```python
from build123d import *
from build123d import SkipClean  # not in build123d's __all__

# Parameters (mm, degrees)
F0_R          = 31.75
F1_DEPTH      = 2.54
F2_R          = 27.305
F2_R_2        = 22.225
F2_R_3        = 6.985
F3_DEPTH      = 5.08
F4_R          = 4.1275
F5_DEPTH      = 25.4
F5_DEPTH_BACK = 96
F7_DEPTH      = 25.4
F7_DEPTH_BACK = 5.081
F8_T1_DEPTH   = 2.54
F10_DEPTH     = 25.4


# Not quite as in the source:
# - a fillet or chamfer that OpenCascade refuses, or shapes differently, is made with other operations: its cross-section is extruded or revolved along the edge and cut away or added
# - an extrude ends at something that could not be found from the text; its depth is read off the source's solid


with BuildPart() as f1:
    # F0 (on Top) → F1 (new body)
    with BuildSketch(Plane.XY):
        Circle(F0_R)
    extrude(amount=F1_DEPTH)

    # F2 (on face) → F3 (join)
    with BuildSketch(Plane.XY.offset(2.54)):
        Circle(F2_R)
        Circle(F2_R_2, mode=Mode.SUBTRACT)
        Circle(F2_R_3)
    extrude(amount=F3_DEPTH)

    # F4 (on face) → F5 (cut, two sides)
    with BuildSketch(Plane.XY.offset(7.62)) as f5_sk:
        Circle(F4_R)
    extrude(amount=-F5_DEPTH, mode=Mode.SUBTRACT)
    extrude(f5_sk.sketch, amount=F5_DEPTH_BACK, mode=Mode.SUBTRACT)

    # F6 (on face) → F7 (cut, two sides)
    with BuildSketch(Plane.XY.offset(2.54)) as f7_sk:
        with BuildLine():
            Line((3.175, 21.9970452561), (3.175, 6.2217039467))
            ThreePointArc((3.175, 6.2217039467), (5.956828015, 3.6477972806), (6.985, 0))
            ThreePointArc((6.985, 0), (6.9826630272, -0.1806711053), (6.9756536726, -0.3612213163))
            Line((6.9756536726, -0.3612213163), (20.6375, -8.248891971))
            ThreePointArc((20.6375, -8.248891971), (21.8245167472, -4.2001302063), (22.225, 0))
            ThreePointArc((22.225, 0), (16.8005208253, 14.5496778315), (3.175, 21.9970452561))
        make_face()
        with BuildLine():
            Line((17.4625, -13.7481532851), (3.8006536726, -5.8604826304))
            ThreePointArc((3.8006536726, -5.8604826304), (0, -6.985), (-3.8006536726, -5.8604826304))
            Line((-3.8006536726, -5.8604826304), (-17.4625, -13.7481532851))
            ThreePointArc((-17.4625, -13.7481532851), (0, -22.225), (17.4625, -13.7481532851))
        make_face()
        with BuildLine():
            ThreePointArc((-6.9756536726, -0.3612213163), (-6.0491874454, 3.4925), (-3.175, 6.2217039467))
            Line((-3.175, 6.2217039467), (-3.175, 21.9970452561))
            ThreePointArc((-3.175, 21.9970452561), (-19.2474145991, 11.1125), (-20.6375, -8.248891971))
            Line((-20.6375, -8.248891971), (-6.9756536726, -0.3612213163))
        make_face()
    with SkipClean():  # cleaning this boolean's faces spoils the solid; the shape is the same uncleaned
        extrude(amount=-F7_DEPTH, mode=Mode.SUBTRACT)
        extrude(f7_sk.sketch, amount=F7_DEPTH_BACK, mode=Mode.SUBTRACT)

    # F8: fillet of radius 1.5875 on 18 edges, made by hand

    # F8_s2 → F8_t1 (join)
    with BuildSketch(Plane.XY):
        with BuildLine():
            ThreePointArc((16.1634751393, -15.2542681378), (16.5796979287, -13.9347220137), (15.8026912008, -12.7898622281))
            Line((15.8026912008, -12.7898622281), (17.4625, -13.7481532851))
            ThreePointArc((17.4625, -13.7481532851), (16.829843924, -14.515749326), (16.1634751393, -15.2542681378))
        make_face()
        with BuildLine():
            ThreePointArc((18.9776912008, -7.290600914), (20.3576722229, -7.3910785865), (21.2923212932, -6.3708460152))
            ThreePointArc((21.2923212932, -6.3708460152), (20.9859296333, -7.3171977169), (20.6375, -8.248891971))
            Line((20.6375, -8.248891971), (18.9776912008, -7.290600914))
        make_face()
        with BuildLine():
            ThreePointArc((3.175, 20.0804631421), (3.7779742942, 21.3258006002), (5.1288461538, 21.625114153))
            ThreePointArc((5.1288461538, 21.625114153), (4.1560857093, 21.8329470429), (3.175, 21.9970452561))
            Line((3.175, 21.9970452561), (3.175, 20.0804631421))
        make_face()
        with BuildLine():
            ThreePointArc((-3.175, 20.0804631421), (-3.7779742942, 21.3258006002), (-5.1288461538, 21.625114153))
            ThreePointArc((-5.1288461538, 21.625114153), (-4.1560857093, 21.8329470429), (-3.175, 21.9970452561))
            Line((-3.175, 21.9970452561), (-3.175, 20.0804631421))
        make_face()
        with BuildLine():
            ThreePointArc((-18.9776912008, -7.290600914), (-20.3576722229, -7.3910785865), (-21.2923212932, -6.3708460152))
            ThreePointArc((-21.2923212932, -6.3708460152), (-20.9859296333, -7.3171977169), (-20.6375, -8.248891971))
            Line((-20.6375, -8.248891971), (-18.9776912008, -7.290600914))
        make_face()
        with BuildLine():
            ThreePointArc((-16.1634751393, -15.2542681378), (-16.5796979287, -13.9347220137), (-15.8026912008, -12.7898622281))
            Line((-15.8026912008, -12.7898622281), (-17.4625, -13.7481532851))
            ThreePointArc((-17.4625, -13.7481532851), (-16.829843924, -14.515749326), (-16.1634751393, -15.2542681378))
        make_face()
        with BuildLine():
            ThreePointArc((4.5854055152, -6.3135593179), (3.8435830552, -6.1017241554), (3.0894970865, -6.2646015638))
            ThreePointArc((3.0894970865, -6.2646015638), (3.4509958561, -6.0729607772), (3.8006536726, -5.8604826304))
            Line((3.8006536726, -5.8604826304), (4.5854055152, -6.3135593179))
        make_face()
        with BuildLine():
            ThreePointArc((-3.0894970865, -6.2646015638), (-3.8435830552, -6.1017241554), (-4.5854055152, -6.3135593179))
            Line((-4.5854055152, -6.3135593179), (-3.8006536726, -5.8604826304))
            ThreePointArc((-3.8006536726, -5.8604826304), (-3.4509958561, -6.0729607772), (-3.0894970865, -6.2646015638))
        make_face()
        with BuildLine():
            ThreePointArc((-7.7604055152, -0.8142980039), (-7.2060396531, -0.2777784896), (-6.970052642, 0.4567178201))
            ThreePointArc((-6.970052642, 0.4567178201), (-6.9848362373, 0.0478303088), (-6.9756536726, -0.3612213163))
            Line((-6.9756536726, -0.3612213163), (-7.7604055152, -0.8142980039))
        make_face()
        with BuildLine():
            ThreePointArc((-3.8805555556, 5.8078837437), (-3.3624565979, 6.379502645), (-3.175, 7.1278573218))
            Line((-3.175, 7.1278573218), (-3.175, 6.2217039467))
            ThreePointArc((-3.175, 6.2217039467), (-3.5338403812, 6.0251304683), (-3.8805555556, 5.8078837437))
        make_face()
        with BuildLine():
            ThreePointArc((3.175, 7.1278573218), (3.3624565979, 6.379502645), (3.8805555556, 5.8078837437))
            ThreePointArc((3.8805555556, 5.8078837437), (3.5338403812, 6.0251304683), (3.175, 6.2217039467))
            Line((3.175, 6.2217039467), (3.175, 7.1278573218))
        make_face()
        with BuildLine():
            ThreePointArc((6.970052642, 0.4567178201), (7.2060396531, -0.2777784896), (7.7604055152, -0.8142980039))
            Line((7.7604055152, -0.8142980039), (6.9756536726, -0.3612213163))
            ThreePointArc((6.9756536726, -0.3612213163), (6.9848362373, 0.0478303088), (6.970052642, 0.4567178201))
        make_face()
    with SkipClean():  # cleaning this boolean's faces spoils the solid; the shape is the same uncleaned
        extrude(amount=F8_T1_DEPTH)

    # F9 (on face) → F10 (cut)
    with BuildSketch(Plane.XY.offset(7.62)):
        with BuildLine():
            ThreePointArc((27.305, 0), (23.6468236503, 13.6525), (13.6525, 23.6468236503))
            Line((13.6525, 23.6468236503), (11.1125, 19.2474145991))
            ThreePointArc((11.1125, 19.2474145991), (19.2474145991, 11.1125), (22.225, 0))
            Line((22.225, 0), (27.305, 0))
        make_face()
        with BuildLine():
            Line((-11.1125, -19.2474145991), (-13.6525, -23.6468236503))
            ThreePointArc((-13.6525, -23.6468236503), (0, -27.305), (13.6525, -23.6468236503))
            Line((13.6525, -23.6468236503), (11.1125, -19.2474145991))
            ThreePointArc((11.1125, -19.2474145991), (0, -22.225), (-11.1125, -19.2474145991))
        make_face()
        with BuildLine():
            ThreePointArc((-22.225, 0), (-19.2474145991, 11.1125), (-11.1125, 19.2474145991))
            Line((-11.1125, 19.2474145991), (-13.6525, 23.6468236503))
            ThreePointArc((-13.6525, 23.6468236503), (-23.6468236503, 13.6525), (-27.305, 0))
            Line((-27.305, 0), (-22.225, 0))
        make_face()
    with SkipClean():  # cleaning this boolean's faces spoils the solid; the shape is the same uncleaned
        extrude(amount=-F10_DEPTH, mode=Mode.SUBTRACT)


solid = f1.part
```
The model under review builds one solid part; all positions refer to its coordinate system, in mm. A direction names the side the tool comes from. Round coordinates to 2 decimals unless told otherwise and drop trailing zeros. Write each loop counter-clockwise with the first axis right and the second up, starting at its lowest first coordinate (ties: lowest second). Pieces come first, ordered by that corner, then holes. Notation, with made-up numbers: (42.5, -21.75) - (49.5, -21.75) arc R9 ccw to (49.5, -14.75) - close; hole circle Ø1 at (16.5, 13.25). An arc over 180 degrees is marked (long way). One line per question, with ' | ' between items.
Item 1: To check wall thickness, follow probe 1 along Y at (x, z) = (0, 4) (1 decimal); probe 2 along Y at (x, z) = (2, 3.75); probe 3 along X at (y, z) = (19.5, 1.75) (3 decimals). State the ranges of each line that lie inside material, in increasing order.
Resolved:
probe 1: y = -7 to -4.1, 4.1 to 7, 22.2 to 27.3 | probe 2: y = -6.69 to -3.61, 3.61 to 6.69, 22.13 to 27.23 | probe 3: x = -25.056 to -19.113, -11.258 to -10.663, -3.175 to 3.175, 10.663 to 11.258, 19.113 to 25.056
Item 2: For P1, Ø2, axis at x = -7.5, z = 2.5, coming from the -Y side; P2, Ø12.5, axis at x = 11, y = -10.5, coming from the +Z side; P3, Ø1, axis at x = -24.5, z = 4.5, coming from the +Y side; P4, Ø8, axis at x = 12, y = 6, coming from the +Z side, all flat-tipped, find the tip position at first contact; note any pin that passes through.
Resolved:
P1: stops at y = -31.08 | P2: stops at z = 2.54 | P3: stops at y = 0 | P4: passes through
Item 3: Add section A-A, the plane z = 4.25. State how many separate pieces and enclosed holes the cut face has, then the cut area to 3 significant figures.
Resolved:
separate pieces: 4 | enclosed holes: 1 | area: 495 mm2
Item 4: For faces 1 (the face through (0, -5, 7.62)), 2 (the face through (0, 14, 2.54)), 3 (the face through (25, 0, 4)), list the 3-axis set-ups (+Z, -Z, +X, -X, +Y, -Y) from which the entire face can be reached by the end or side of a thin tool; tool diameter is ignored.
Resolved:
face 1: +Z, +X, -X, +Y, -Y | face 2: +Z | face 3: +Z, -Z
Item 5: Add section D-D, the plane x = -25. Give the boundary of the cut face in (y, z), then the cut area to 3 significant figures.
Resolved:
outline: (-19.57, 0) - (0, 0) - (0, 7.62) - (-10.98, 7.62) - (-10.98, 2.54) - (-19.57, 2.54) - close; (10.98, 0) - (19.57, 0) - (19.57, 2.54) - (10.98, 2.54) - close | area: 127 mm2
Item 6: Add section C-C, the plane y = -10. Give the boundary of the cut face in (x, z), then the cut area to 3 significant figures.
Resolved:
outline: (-30.13, 0) - (-10.97, 0) - (-10.97, 2.54) - (-19.85, 2.54) - (-19.85, 7.62) - (-25.41, 7.62) - (-25.41, 2.54) - (-30.13, 2.54) - close; (10.97, 0) - (30.13, 0) - (30.13, 2.54) - (25.41, 2.54) - (25.41, 7.62) - (19.85, 7.62) - (19.85, 2.54) - (10.97, 2.54) - close | area: 154 mm2
Item 7: The part is to be moulded in two halves that separate along Y. For faces 4 (the face through (-6.883, -30.995, 1.252)), 5 (the face through (16.58, -13.95, 1.25)), 6 (the face through (-16.58, -13.95, 1.25)), 7 (the face through (-20, -13, 7.62)), say which applies: pulls with the +Y half, pulls with the -Y half, needs draft (parallel to the pull), parting line crosses it, or undercut.
Resolved:
face 4: parting line crosses it | face 5: undercut | face 6: undercut | face 7: needs draft
